from build123d import *

# Parameters (mm, degrees)
SWEEP1_PROFILE_R     = 15
CHAMFER1_SIZE        = 0.5
CHAMFER1_SIZE_2      = 0.589255651
CUT_SWEEP1_PROFILE_R = 10
SKETCH39_R           = 10.414
CUT_EXTRUDE1_DEPTH   = 12.790226
FILLET1_R            = 2
CUT_EXTRUDE3_REACH   = 209.074
SKETCH66_R           = 19
SKETCH67_R           = 10
CUT_EXTRUDE4_DEPTH   = 193.040325543


with BuildPart() as part:
    # Sketch1 → Revolve1 (revolve)
    with BuildSketch(Plane.XY, mode=Mode.PRIVATE) as revolve1_sk:
        with BuildLine():
            Line((0, 0), (32.5, 0))
            Line((32.5, 0), (32.5, 7))
            Line((32.5, 7), (29.5, 7))
            ThreePointArc((29.5, 7), (24.607160678, 12.840669622), (22, 20))
            Line((22, 20), (25, 23))
            ThreePointArc((25, 23), (22.781598043, 26.192113447), (22, 30))
            Line((22, 30), (22, 128))
            ThreePointArc((22, 128), (22.769750529, 132.74341649), (25, 137))
            Line((25, 137), (22, 140))
            Line((22, 140), (0, 140))
            Line((0, 140), (0, 0))
        make_face()
    revolve(revolve1_sk.sketch.rotate(Axis((0, 140, 0), (0, -1, 0)), 90), axis=Axis((0, 140, 0), (0, -1, 0)))

    # Sweep1: sweep along a path in Sketch3
    with BuildLine(Plane.XY) as sweep1_path:
        Line((0, 105), (97, 105))
        ThreePointArc((97, 105), (105.059494125, 102.650871687), (110.594616806, 96.339273926))
    # Sweep1 profile (on start of the path) → Sweep1 (sweep)
    with BuildSketch(Plane(origin=(0, 105, 0), x_dir=(0, 1, 0), z_dir=(1, 0, 0))):
        Circle(SWEEP1_PROFILE_R)
    sweep(path=sweep1_path.line)

    # Sketch16 → Revolve3 (revolve)
    with BuildSketch(Plane.XY, mode=Mode.PRIVATE) as revolve3_sk:
        with BuildLine():
            Line((116, 84.747392258), (126.875693444, 89.818811398))
            Line((126.875693444, 89.818811398), (124.762602136, 94.350350334))
            Line((124.762602136, 94.350350334), (127.650557609, 98.620990158))
            ThreePointArc((127.650557609, 98.620990158), (125.644403351, 100.414758676), (124.189233611, 102.678547852))
            Line((124.189233611, 102.678547852), (110.594616806, 96.339273926))
            Line((110.594616806, 96.339273926), (116, 84.747392258))
        make_face()
    revolve(revolve3_sk.sketch.rotate(Axis((110.594616806, 96.339273926, 0), (0.4226182617406933, -0.9063077870366529, 0)), 180), axis=Axis((110.594616806, 96.339273926, 0), (0.4226182617406933, -0.9063077870366529, 0)))

    # Chamfer1
    # the kernel refuses this chamfer: 0.589255651, 0.5, 0.488240397 mm, written as the material it takes off along each edge
    with BuildSketch(Plane(origin=(0, 23, 0), x_dir=(0, 0, 1), z_dir=(1, 0, 0))) as chamfer1_piece_1:
        with BuildLine():
            Line((25 - CHAMFER1_SIZE * 0.707106781187, CHAMFER1_SIZE * 0.707106781187), (24.646446609, -0.35462907))
            ThreePointArc((24.646446609, -0.35462907), (24.815923099, -0.18004714), (25, 0))
            Line((25, 0), (25 - CHAMFER1_SIZE * 0.707106781187, CHAMFER1_SIZE * 0.707106781187))
        make_face()
    revolve(axis=Axis((0, 23, 0), (0, -1, 0)), mode=Mode.SUBTRACT)
    with BuildSketch(Plane(origin=(112.766965477, 91.680657166, 0), x_dir=(-0.9063077870366528, -0.42261826174069334, 0), z_dir=(0, 0, 1))) as chamfer1_piece_2:
        with BuildLine():
            Line((16.169745555, -0.446963708), (16.422226913 - CHAMFER1_SIZE * 0.857777308691, CHAMFER1_SIZE * 0.514021486608))
            Line((16.422226913 - CHAMFER1_SIZE * 0.857777308691, CHAMFER1_SIZE * 0.514021486608), (16.422226913, 0))
            ThreePointArc((16.422226913, 0), (16.289550416, -0.228181881), (16.169745555, -0.446963708))
        make_face()
    revolve(axis=Axis((112.766965477, 91.680657166, 0), (0.4226182617406933, -0.9063077870366529, 0)), mode=Mode.SUBTRACT)
    with BuildSketch(Plane(origin=(0, 137, 0), x_dir=(0, 0, 1), z_dir=(1, 0, 0))) as chamfer1_piece_3:
        with BuildLine():
            Line((24.701725164, 0.412076149), (25 - CHAMFER1_SIZE_2 * 0.707106781173, -CHAMFER1_SIZE_2 * 0.707106781173))
            Line((25 - CHAMFER1_SIZE_2 * 0.707106781173, -CHAMFER1_SIZE_2 * 0.707106781173), (25, 0))
            ThreePointArc((25, 0), (24.844145725, 0.211643678), (24.701725164, 0.412076149))
        make_face()
    revolve(axis=Axis((0, 137, 0), (0, -1, 0)), mode=Mode.SUBTRACT)

    # Cut-Sweep1: sweep along a path in Sketch3<3>
    with BuildLine(Plane.XY) as cut_sweep1_path:
        Line((0, 105), (97, 105))
        ThreePointArc((97, 105), (105.059494125, 102.650871687), (110.594616806, 96.339273926))
    # Cut-Sweep1 profile (on start of the path) → Cut-Sweep1 (sweep, cut)
    with BuildSketch(Plane(origin=(0, 105, 0), x_dir=(0, 1, 0), z_dir=(1, 0, 0))):
        Circle(CUT_SWEEP1_PROFILE_R)
    sweep(path=cut_sweep1_path.line, mode=Mode.SUBTRACT)

    # Sketch39 → Cut-Extrude1 (cut)
    with BuildSketch(Plane(origin=(-11.741815816, 25.180405276, 0), x_dir=(-0.9063077870366528, -0.4226182617406934, 0), z_dir=(0.42261826174069334, -0.9063077870366527, 0))):
        with Locations(Location((-140.947498899, 0, 0), (0, 0, 180))):
            Circle(SKETCH39_R)
    extrude(amount=-CUT_EXTRUDE1_DEPTH, mode=Mode.SUBTRACT)

    # Fillet1
    fillet1_edges = [part.edges().sort_by_distance(p)[0] for p in [
        (22, 90, 0),
    ]]
    fillet(fillet1_edges, radius=FILLET1_R)

    # Sketch65 → Revolve4 (revolve)
    with BuildSketch(Plane.XY):
        with BuildLine():
            Line((20, 140), (17, 140))
            ThreePointArc((17, 140), (12.02081528, 152.02081528), (0, 157))
            Line((0, 157), (0, 160))
            ThreePointArc((0, 160), (14.142135624, 154.142135624), (20, 140))
        make_face()
    revolve(axis=Axis((0, 160, 0), (0, -1, 0)))

    # Cut-Extrude3: up to this face of the body (flat: up to its plane)
    cut_extrude3_end = Plane(part.part.faces().sort_by_distance((0, 140, -21.377746033))[0])
    # Sketch66 → Cut-Extrude3 (cut, up to the picked face)
    with BuildSketch(Plane.XZ, mode=Mode.PRIVATE) as cut_extrude3_sk1:
        with Locations(Location((0, 0, 0), (0, 0, 270))):
            Circle(SKETCH66_R)
    cut_extrude3_tool1 = split(extrude(cut_extrude3_sk1.sketch, amount=-CUT_EXTRUDE3_REACH, mode=Mode.PRIVATE), bisect_by=cut_extrude3_end, keep=Keep.BOTH, mode=Mode.PRIVATE)
    add(cut_extrude3_tool1.solids().sort_by(Axis((0, 0, 0), (0, 1, 0)))[0], mode=Mode.SUBTRACT)

    # Sketch67 → Cut-Extrude4 (cut, through all)
    with BuildSketch(Plane(origin=(0, 140, 0), x_dir=(1, 0, 0), z_dir=(0, 1, 0))):
        with Locations(Location((0, 0, 0), (0, 0, 90))):
            Circle(SKETCH67_R)
    extrude(amount=CUT_EXTRUDE4_DEPTH, mode=Mode.SUBTRACT)


solid = part.part
Read the model definition and answer for the solid it produces. Units are mm, in the model's axes. A direction names the side the tool comes from. Give positions to 0.01 mm unless a question says otherwise; leave off trailing zeros. Write each loop counter-clockwise with the first axis right and the second up, starting at its lowest first coordinate (ties: lowest second). Pieces come first, ordered by that corner, then holes. Notation, with made-up numbers: (-14.5, 34.5) -> (28.5, 34.5) arc R23 cw to (28.5, 63.5) -> close; hole circle Ø7 at (56, 29.25). An arc over 180 degrees is marked (long way). Answer as a JSON object with one key per item and string values. Group by question number.
1) Consider L1, parallel to X at y = 93, z = 0; L2, parallel to X at y = 92.5, z = 0; L3, parallel to Y at x = 46, z = 0. Determine where each line is inside the solid, lowest interval first. Write a range as from..to.
2) A tool of negligible diameter and unlimited length cuts with its end or side. For faces 1 (the flat face through (115.9, 84.7, -10.7)), 2 (the cylindrical face through (-18.548, 69.02, 4.119)), 3 (the cylindrical face through (9.76, 155.51, 2.17)), 4 (the flat face through (18, 140, 10)), 5 (the conical face through (-6.658, 20.166, 21.142)), from which of +Z, -Z, +X, -X, +Y, -Y can it reach the whole face along a straight path? Write none if from no direction.
3) Find section D-D (z = 4). Count the separate pieces of the cut face and the enclosed holes in it, and give its area (3 significant figures).
4) Find section C-C (x = 47). Write down the section's boundary in (y, z), and give its area (3 significant figures).
5) Find section B-B (y = 10.5). Write down the section's boundary in (x, z), and give its area (3 significant figures).
6) The mould has two halves that part along Z. Classify faces 6 (the cylindrical face through (57, 95, 0)), 7 (the cylindrical face through (-7.4, 23.01, 23.51)), 8 (the flat face through (14, 0, -14)): +Z half, -Z half, draft (parallel to the pull), parting line (faces both ways), or undercut.
7) Each of these flat-tipped pins is pushed along its axis until it touches: P1, Ø2, axis at x = 110, z = 5, coming from the -Y side; P2, Ø11.5, axis at x = -4.5, z = 5.5, coming from the -Y side; P3, Ø1, axis at y = 34, z = -8.5, coming from the -X side; P4, Ø1.5, axis at x = 24, y = 53.5, coming from the +Z side. Where does it stop, or does it pass through?
Values follow:
{
 "1": {"L1": "x = -22..-19, 19..101, 123.64..125.39", "L2": "x = -22..-19, 19..101.33, 123.88..125.63", "L3": "y = 90..95, 115..120"},
 "2": {"face 1": "+Z, -Z, +X, -Y", "face 2": "-Y", "face 3": "+Y, -Y", "face 4": "+Y", "face 5": "none"},
 "3": {"separate pieces": "3", "enclosed holes": "0", "area": "2,260 mm2"},
 "4": {"outline": "circle Ø30 at (105, 0); hole circle Ø20 at (105, 0)", "area": "393 mm2"},
 "5": {"outline": "circle Ø52.33 at (0, 0); hole circle Ø38 at (0, 0)", "area": "1,020 mm2"},
 "6": {"face 6": "undercut", "face 7": "parting line", "face 8": "draft"},
 "7": {"P1": "stops at y = 108.73", "P2": "stops at y = 151.12", "P3": "stops at x = -20.49", "P4": "passes through"}
}
